Autodesk Inventor part; units mm, degrees
ref_plane "YZ Plane" through (0, 0, 0) normal (1, 0, 0) x (0, 1, 0)
ref_plane "XZ Plane" through (0, 0, 0) normal (0, 1, 0) x (-1, 0, 0)
ref_plane "XY Plane" through (0, 0, 0) normal (0, 0, 1) x (1, 0, 0)
sketch "Sketch1" plane through (0, 0, 0) normal (0, 0, 1) x (1, 0, 0)
  line L0 (0, 0) -> (0, 50.8)
  arc A0 (88.9, 50.8) -> (0, 50.8) centre (44.45, 50.8) ccw
  line L1 (88.9, 50.8) -> (88.9, 0)
  line L2 (89.6874, 0) -> (89.6874, 50.8)
  arc A1 (89.6874, 50.8) -> (-0.7874, 50.8) centre (44.45, 50.8) ccw
  line L3 (-0.7874, 50.8) -> (-0.7874, 0)
  line L4 (-0.7874, 50.8) -> (50.0126, 50.8) construction
  line L5 (88.9, 0) -> (88.8999, -101.6)
  line L6 (89.6874, -1.5875) -> (89.6874, -101.6)
  line L7 (89.6874, -101.6) -> (88.8999, -101.6)
  line L8 (-0.7874, 0) -> (-0.7874, -101.6)
  line L9 (0, 0) -> (-0.0001, -101.6)
  line L10 (-0.0001, -101.6) -> (-0.7874, -101.6)
  line L11 (89.6874, 0) -> (89.6874, -1.5875)
  dimension "d1" = 88.9
  dimension "d2" = 44.45
  dimension "d3" = 50.8
  dimension "d5" = 50.8
  dimension "d6" = 90.4748
  dimension "d7" = 45.2374
  dimension "d8" = 50.8
  dimension "d9" = 90
  dimension "d30" = 101.6
  dimension "d32" = 101.6
extrude "Extrusion1" add sketch "Sketch1" along normal blind 12.7
hole "Hole1" at (89.6874, 12.7, 6.35) direction (-1, 0, 0) diameter 6.35 end through all
hole "Hole2" at (89.6874, 38.1, 6.35) direction (-1, 0, 0) diameter 6.35 end through all
sketch "Sketch3" plane through (-0.7874, -101.6, 0) normal (-1, 0, 0) x (0, 0, 1)
  line L0 (0, 101.6) -> (12.7, 101.6)
  line L1 (6.35, 101.6) -> (6.35, 88.9)
  line L2 (6.35, 88.9) -> (6.35, 63.5)
  dimension "d36" = 12.7
  dimension "d37" = 25.4
sketch "Sketch4" plane through (-0.7874, 0, 0) normal (-1, 0, 0) x (0, 0, 1)
  circle A0 centre (6.35, 38.1) radius 3.175
  circle A1 centre (6.35, 12.7) radius 3.175
  line L0 (0, 50.8) -> (0, 0)
  line L1 (0, 0) -> (12.7, 0)
  line L2 (12.7, 50.8) -> (12.7, 0)
  line L3 (0, 50.8) -> (12.7, 50.8)
  dimension "d34" = 12.7
hole "Hole3" at (-0.7874, -12.7, 6.35) direction (1, 0, 0) diameter 6.35 end through all
sketch "Sketch5" plane through (-0.7874, -101.6, 0) normal (-1, 0, 0) x (0, 0, 1)
  circle A0 centre (6.35, 88.9) radius 3.175
  line L0 (0, 0) -> (12.7, 0)
  line L1 (0, 101.6) -> (12.7, 101.6)
  line L2 (6.35, 88.9) -> (6.35, 63.5)
  line L3 (6.35, 88.9) -> (31.75, 88.9) construction
  line L4 (6.35, 63.5) -> (6.35, 38.1)
  line L5 (6.35, 38.1) -> (6.35, 12.7)
  dimension "d45" = 25.4
  dimension "d46" = 90
  dimension "d47" = 25.4
  dimension "d48" = 25.4
hole "Hole4" at (-0.7874, -38.1, 6.35) direction (1, 0, 0) diameter 6.35 end through all
sketch "Sketch6" plane through (-0.7874, -101.6, 0) normal (-1, 0, 0) x (0, 0, 1)
  circle A0 centre (6.35, 63.5) radius 3.175
  line L0 (0, 101.6) -> (12.7, 101.6)
  line L1 (6.35, 63.5) -> (6.35, 38.1)
  dimension "d56" = 25.4
hole "Hole5" at (-0.7874, -63.5, 6.35) direction (1, 0, 0) diameter 6.35 end through all
sketch "Sketch7" plane through (-0.7874, -101.6, 0) normal (-1, 0, 0) x (0, 0, 1)
  circle A0 centre (6.35, 38.1) radius 3.175
  line L0 (0, 101.6) -> (12.7, 101.6)
  line L1 (6.35, 38.1) -> (6.35, 12.7)
  dimension "d64" = 25.4
hole "Hole6" at (-0.7874, -88.9, 6.35) direction (1, 0, 0) diameter 6.35 end through all
properties part number "Strap"
Build history of the part. All positions in model axes, mm. Round coordinates to 2 decimals unless told otherwise and drop trailing zeros. Write each loop counter-clockwise with the first axis right and the second up, starting at its lowest first coordinate (ties: lowest second). Pieces come first, ordered by that corner, then holes. Notation, with made-up numbers: M 29,56.5 L 73,56.5 A15 ccw 73,85.5 Z; hole C 50,39.25 d6. An arc over 180 degrees is marked long. Use CSV: the item, a comma, the result in double quotes.
1. Saw through at A-A (y = -3). Give the cut face in (x, z).
Reply:
outline,"M -0.79,0 L 0,0 L 0,12.7 L -0.79,12.7 Z; M 88.9,0 L 89.69,0 L 89.69,12.7 L 88.9,12.7 Z"
2. Saw through at D-D (x = 9.5). Give the cut face in (y, z), plus the area to 3 significant figures.
Reply:
outline,"M 78.26,0 L 79.52,0 L 79.52,12.7 L 78.26,12.7 Z"
area,"16.0 mm²"
3. Saw through at C-C (z = 6.35). State how many separate pieces and enclosed holes the cut face has, plus the area to 3 significant figures.
Reply:
separate pieces,"13"
enclosed holes,"0"
area,"291 mm²"
4. Saw through at B-B (y = -38.1). Give the cut face in (x, z) (3 decimals), plus the area to 4 significant figures.
Reply:
outline,"M -0.787,0 L 0,0 L 0,3.175 L -0.787,3.175 Z; M -0.787,9.525 L 0,9.525 L 0,12.7 L -0.787,12.7 Z; M 88.9,0 L 89.687,0 L 89.687,3.175 L 88.9,3.175 Z; M 88.9,9.525 L 89.687,9.525 L 89.687,12.7 L 88.9,12.7 Z"
area,"10.00 mm²"
5. Flat gauge pins, fed straight in: pin 1 (2 mm diameter, centred on x = 17, z = 5, fed in from +Y); pin 2 (1.5 mm diameter, centred on x = 8.5, z = 7, fed in from -Y); pin 3 (1 mm diameter, centred on x = 74, z = 2.5, fed in from +Y). Where does each tip first touch, or does it go through?
Reply:
pin 1,"stops at y = 87.5"
pin 2,"stops at y = 75.88"
pin 3,"stops at y = 85.48"
6. Two-plate mould, pull along Y, no slides. Class faces 1 (the face through (-0.39, -36.17, 3.83)), 2 (the face through (43.455, 96.026, 6.261)), 3 (the face through (89.687, -26, 6)), 4 (the face through (89.288, 35.423, 4.643)): +Y half, -Y half, draft (parallel to the pull), parting line (faces both ways), or undercut.
Reply:
face 1,"undercut"
face 2,"+Y half"
face 3,"draft"
face 4,"undercut"
7. Wall check: probe 1 along X at (y, z) = (-66, 8.5); probe 2 along Z at (x, y) = (89.35, -88.9) (3 decimals); probe 3 along X at (y, z) = (84.5, 3.75). Give the ranges that are in metal, low to high. Write a range as from..to.
Reply:
probe 1,"x = -0.79..0, 88.9..89.69"
probe 2,"z = 0..3.175, 9.525..12.7"
probe 3,"x = 14.27..15.47, 73.43..74.63"
